from build123d import *

# Parameters (mm, degrees)
F0_R     = 2.5
F1_DEPTH = 55
F2_R     = 4.2
F3_DEPTH = 5
F4_R     = 5
F5_DEPTH = 1


with BuildPart() as f1:
    # F0 (on Top) → F1 (new body)
    with BuildSketch(Plane.XY):
        Circle(F0_R)
    extrude(amount=-F1_DEPTH)

    # F2 (on Top) → F3 (join)
    with BuildSketch(Plane.XY):
        Circle(F2_R)
    extrude(amount=F3_DEPTH)

    # F4 (on Top) → F5 (join)
    with BuildSketch(Plane.XY):
        Circle(F4_R)
    extrude(amount=-F5_DEPTH)


solid = f1.part
Verification items for the finished model (mm, model axes). A direction names the side the tool comes from. Give positions to 0.01 mm unless a question says otherwise; leave off trailing zeros. Write each loop counter-clockwise with the first axis right and the second up, starting at its lowest first coordinate (ties: lowest second). Pieces come first, ordered by that corner, then holes. Notation, with made-up numbers: (89.25, 16) - (148.25, 16) arc R14 ccw to (148.25, 28) - close; hole circle Ø4 at (-36, -38.5). An arc over 180 degrees is marked (long way). Answer as CSV lines item,"result". Start each with the question number.
1. Sectioned sample at B-B (x = 1.25). Record the boundary of the cut face in (y, z), then the cut area to 3 significant figures.
2. Sectioned sample at C-C (z = -14). Record the boundary of the cut face in (x, y).
3. Sectioned sample at A-A (y = 0). Record the boundary of the cut face in (x, z).
4. Set-up check for faces 1 (the face through (0, 0, -55)), 2 (the face through (-0.54, -2.44, -27.62)), 3 (the face through (4.006, 1.262, 2.465)): record each of +Z, -Z, +X, -X, +Y, -Y from which the full face is reachable in a straight line by a thin tool's end or side.
5. Thickness scan on line 1 (Z direction, x = 1.5, y = -2.5); line 2 (X direction, y = -0.25, z = -21.5); line 3 (Z direction, x = -4.5, y = 0.5). Record the ranges inside material, lowest first.
6. Depth check by flat-ended pin: pin 1 (3 mm diameter, centred on x = 3, z = -8, fed in from -Y); pin 2 (2 mm diameter, centred on y = -3, z = -16.5, fed in from +X); pin 3 (6 mm diameter, centred on x = -1.5, z = -47.5, fed in from +Y). Enter the tip coordinate at first touch or a pass-through.
Derived:
1,outline,"(-4.84, -1) - (-2.17, -1) - (-2.17, -55) - (2.17, -55) - (2.17, -1) - (4.84, -1) - (4.84, 0) - (4.01, 0) - (4.01, 5) - (-4.01, 5) - (-4.01, 0) - (-4.84, 0) - close"
1,area,"284 mm²"
2,outline,"circle Ø5 at (0, 0)"
3,outline,"(-5, -1) - (-2.5, -1) - (-2.5, -55) - (2.5, -55) - (2.5, -1) - (5, -1) - (5, 0) - (4.2, 0) - (4.2, 5) - (-4.2, 5) - (-4.2, 0) - (-5, 0) - close"
4,face 1,"-Z, +X, -X, +Y, -Y"
4,face 2,"-Z"
4,face 3,"+Z"
5,line 1,"-1 to 5"
5,line 2,"-2.49 to 2.49"
5,line 3,"-1 to 0"
6,pin 1,"y = -2"
6,pin 2,"x = 1.5"
6,pin 3,"y = 2.5"
